Solid Edge part; units mm, degrees
sketch "Sketch1" plane through (0, 0, 0) normal (0, -1, 0) x (1, 0, 0)
  line L0 (3.5, 2.0207) -> (0, 4.0415)
  line L1 (0, 4.0415) -> (-3.5, 2.0207)
  line L2 (-3.5, 2.0207) -> (-3.5, -2.0207)
  line L3 (-3.5, -2.0207) -> (0, -4.0415)
  line L4 (0, -4.0415) -> (3.5, -2.0207)
  line L5 (3.5, -2.0207) -> (3.5, 2.0207)
extrude "Protrusion1" add sketch "Sketch1" along normal mid plane 2.2
sketch "Sketch2" plane through (0, 0, 0) normal (1, 0, 0) x (0, 1, 0)
  line L0 (-1.1, 2.95) -> (-0.8075, 4.0415)
revolve "RevolvedCutout1" cut sketch "Sketch2" angle 360 about axis through (0, 0, 0) along (0, -1, 0) material side at (0, -1.002, 3.5087)
mirror "Mirror1" about plane through (0, 0, 0) normal (0, -1, 0) of "RevolvedCutout1"
hole "孔_7" at (0, -1.1, 0) direction (0, 1, 0) diameter 3.242 end up to next start chamfer 0.4 start chamfer angle 60 end chamfer 0.4 end chamfer angle 60
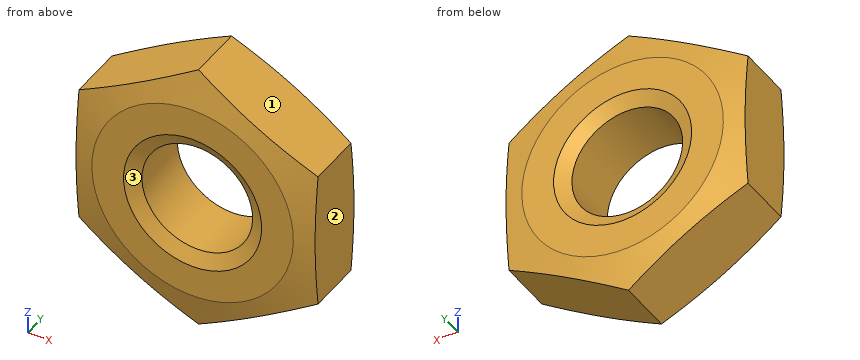
Verification items for the finished model (mm, model axes). Face numbers are marked on the shaded views. Give positions to 0.01 mm unless a question says otherwise; leave off trailing zeros. Loops run counter-clockwise (first coordinate to the right, second up) from the corner with the lowest first, then second, coordinate; pieces in that order, holes last. Notation, with made-up numbers: M 27.5,54 L 52.5,54 A15 cw 52.5,67 Z; hole C 53,43.25 d4. An arc over 180 degrees is marked long. Return JSON: item names as keys, results as strings.
1) Mould release check, pull along Z, two halves, no side actions. Record for the marked faces 1, 2 and 3: released by +Z, released by -Z, zero draft, split by the parting line, or undercut.
Findings:
{"face 1": "released by +Z", "face 2": "zero draft", "face 3": "undercut"}
2) Section check B-B, the plane y = -0.2. Enter the section's corners in (x, z).
Findings:
{"outline": "M -3.5,-2.02 L 0,-4.04 L 3.5,-2.02 L 3.5,2.02 L 0,4.04 L -3.5,2.02 Z; hole C 0,0 d3.24"}
3) Material ranges on L1, parallel to X at y = 0.5, z = 0; L2, parallel to Z at x = -0.75, y = -0.7; L3, parallel to Z at x = 1, y = 0.3, recorded low to high. Write a range as [from, to].
Findings:
{"L1": "x = [-3.5, -1.62], [1.62, 3.5]", "L2": "z = [-3.61, -1.44], [1.44, 3.61]", "L3": "z = [-3.46, -1.28], [1.28, 3.46]"}
4) Section check A-A, the plane z = 0. Enter the section's corners in (x, y).
Findings:
{"outline": "M -3.5,-0.95 L -2.95,-1.1 L -2.02,-1.1 L -1.62,-0.87 L -1.62,0.87 L -2.02,1.1 L -2.95,1.1 L -3.5,0.95 Z; M 1.62,-0.87 L 2.02,-1.1 L 2.95,-1.1 L 3.5,-0.95 L 3.5,0.95 L 2.95,1.1 L 2.02,1.1 L 1.62,0.87 Z"}
